Can you work these out from the model? Positions are in its coordinate system, mm. A direction names the side the tool comes from. Round coordinates to 2 decimals unless told otherwise and drop trailing zeros. Loops run counter-clockwise (first coordinate to the right, second up) from the corner with the lowest first, then second, coordinate; pieces in that order, holes last. Notation, with made-up numbers: (67, 43.5) -> (124, 43.5) arc R13 cw to (124, 59.5) -> close; hole circle Ø2 at (87.5, 61.25). An arc over 180 degrees is marked (long way). Use a Markdown table: item, result.
from build123d import *

# Parameters (mm, degrees)
SKETCH1_R                = 3
BOSS_EXTRUDE1_DEPTH      = 2.3
SHELL1_T                 = -1.5
BOSS_EXTRUDE2_DEPTH      = 1.6
BOSS_EXTRUDE2_DEPTH_BACK = 0.4
SKETCH2_R                = 4.5
SKETCH2_R_2              = 3
FILLET4_R                = 0.2


with BuildPart() as part:
    # Sketch1 → Boss-Extrude1 (new body)
    with BuildSketch(Plane(origin=(0, 0, 0), x_dir=(1, 0, 0), z_dir=(0, 1, 0))):
        with Locations(Location((0, 0, 0), (0, 0, 270))):
            Circle(SKETCH1_R)
    extrude(amount=BOSS_EXTRUDE1_DEPTH)

    # Shell1
    shell1_openings = [part.faces().sort_by_distance(p)[0] for p in [
        (0, 2.3, 0),
        (0, 0, 0),
    ]]
    offset(amount=SHELL1_T, openings=shell1_openings, kind=Kind.INTERSECTION)

    # Sketch2 → Boss-Extrude2 (add, two sides: drawn at the far end of the back side and taken through both)
    with BuildSketch(Plane.XZ.offset(-BOSS_EXTRUDE2_DEPTH_BACK)):
        with Locations(Location((0, 0, 0), (0, 0, 270))):
            Circle(SKETCH2_R)
        with Locations(Location((0, 0, 0), (0, 0, 270))):
            Circle(SKETCH2_R_2, mode=Mode.SUBTRACT)
    extrude(amount=BOSS_EXTRUDE2_DEPTH + BOSS_EXTRUDE2_DEPTH_BACK)

    # Fillet4
    fillet4_edges = [part.edges().sort_by_distance(p)[0] for p in [
        (0, 0.4, -3),
        (0, 0, 3),
    ]]
    fillet(fillet4_edges, radius=FILLET4_R)


solid = part.part
1. I want a section at D-D (y = 1.5). Please give me the cut outline in (x, z).
Answer sheet:
| item | result |
|---|---|
| outline | circle Ø6 at (0, 0); hole circle Ø3 at (0, 0) |
2. Will this pin go through, and if not, where does the flat tip stop? pin 1 Ø3 at (x, z) = (-1, 0) entering from -Y.
Answer sheet:
| item | result |
|---|---|
| pin 1 | stops at y = 0 |
3. I want a section at B-B (y = -0.85). Please give me the cut outline in (x, z).
Answer sheet:
| item | result |
|---|---|
| outline | circle Ø9 at (0, 0); hole circle Ø6 at (0, 0) |
4. I want a section at C-C (x = -3.75). Please give me the cut outline in (y, z), plus the area to 3 significant figures.
Answer sheet:
| item | result |
|---|---|
| outline | (-1.6, -2.49) -> (0.4, -2.49) -> (0.4, 2.49) -> (-1.6, 2.49) -> close |
| area | 9.95 mm² |
5. If we mould it in two halves opening along Z, with no side actions, what happens to faces 1 (the cylindrical face through (1.352, -0.586, -4.292)), 2 (the cylindrical face through (0.9, -0.89, -2.86)), 3 (the flat face through (-1.3, 2.3, 1.3))? For each: +Z half, -Z half, draft (parallel to the pull), parting line (faces both ways), or undercut.
Answer sheet:
| item | result |
|---|---|
| face 1 | parting line |
| face 2 | undercut |
| face 3 | draft |
6. Which directions (+Z, -Z, +X, -X, +Y, -Y) give clear straight access to the entire face, cutting with the end or side of a thin tool? Please do faces 4 (the flat face through (-1.2, 0, 1.2)), 5 (the cylindrical face through (0.45, 1.13, 1.43)), 6 (the flat face through (-3, 0.4, -2)).
Answer sheet:
| item | result |
|---|---|
| face 4 | -Y |
| face 5 | +Y, -Y |
| face 6 | +Y |
7. I need wall thicknesses on line 1 (X direction, y = 0.8, z = 0); line 2 (X direction, y = -1, z = 0). Which ranges of each line are inside material? Lowest first, please.
Answer sheet:
| item | result |
|---|---|
| line 1 | x = -3 to -1.5, 1.5 to 3 |
| line 2 | x = -4.5 to -3, 3 to 4.5 |
8. I want a section at A-A (z = 0). Please give me the cut outline in (x, y), plus the area to 3 significant figures.
Answer sheet:
| item | result |
|---|---|
| outline | (-4.5, -1.6) -> (-3, -1.6) -> (-3, -0.2) arc R0.2 cw to (-2.8, 0) -> (-1.5, 0) -> (-1.5, 2.3) -> (-3, 2.3) -> (-3, 0.6) arc R0.2 cw to (-3.2, 0.4) -> (-4.5, 0.4) -> close; (1.5, 0) -> (2.8, 0) arc R0.2 cw to (3, -0.2) -> (3, -1.6) -> (4.5, -1.6) -> (4.5, 0.4) -> (3.2, 0.4) arc R0.2 cw to (3, 0.6) -> (3, 2.3) -> (1.5, 2.3) -> close |
| area | 12.9 mm² |
